Check sheet for the modelled part. Datum: model origin and axes. Units: mm. A direction names the side the tool comes from. Give positions to 0.01 mm unless a question says otherwise; leave off trailing zeros. Loops run counter-clockwise (first coordinate to the right, second up) from the corner with the lowest first, then second, coordinate; pieces in that order, holes last. Notation, with made-up numbers: M 28.25,36 L 37.25,36 A9 ccw 37.25,51 Z; hole C -12,-37 d6. An arc over 180 degrees is marked long. Use one line per item in the form item = value.
from build123d import *

# Parameters (mm, degrees)
SKETCH1_W                = 240
SKETCH1_H                = 240
BOSS_EXTRUDE1_DEPTH      = 20
CUT_EXTRUDE1_DEPTH       = 210.045449604
CUT_EXTRUDE1_DEPTH_BACK  = 210.045449604
SKETCH2_R                = 3.3
SKETCH3_R                = 5.5
CUT_EXTRUDE3_DEPTH       = 6.5
CUT_EXTRUDE4_DEPTH       = 210.045449604
CUT_EXTRUDE4_DEPTH_BACK  = 210.045449604
SKETCH4_R                = 6.75
SKETCH5_R                = 10
CUT_EXTRUDE6_DEPTH       = 13
CUT_EXTRUDE7_DEPTH       = 210.045449604
CUT_EXTRUDE7_DEPTH_BACK  = 210.045449604
SKETCH6_R                = 3.3
SKETCH7_R                = 5.5
CUT_EXTRUDE9_DEPTH       = 6.5
CUT_EXTRUDE10_DEPTH      = 210.045449604
CUT_EXTRUDE10_DEPTH_BACK = 210.045449604
SKETCH8_W                = 30
SKETCH8_H                = 260


with BuildPart() as part:
    # Sketch1 → Boss-Extrude1 (new body)
    with BuildSketch(Plane.XY):
        with Locations((0, -50)):
            Rectangle(SKETCH1_W, SKETCH1_H)
    extrude(amount=BOSS_EXTRUDE1_DEPTH)

    # Sketch2 → Cut-Extrude1 (cut, two sides: drawn at the far end of the back side and taken through both)
    with BuildSketch(Plane.XY.offset(-CUT_EXTRUDE1_DEPTH_BACK)):
        with Locations((-52, -63)):
            Circle(SKETCH2_R)
        with Locations((-52, 63)):
            Circle(SKETCH2_R)
        with Locations((52, -63)):
            Circle(SKETCH2_R)
        with Locations((52, 63)):
            Circle(SKETCH2_R)
    extrude(amount=CUT_EXTRUDE1_DEPTH + CUT_EXTRUDE1_DEPTH_BACK, mode=Mode.SUBTRACT)

    # Sketch3 → Cut-Extrude3 (cut)
    with BuildSketch(Plane.XY.offset(20)):
        with Locations((-52, -63)):
            Circle(SKETCH3_R)
        with Locations((-52, 63)):
            Circle(SKETCH3_R)
        with Locations((52, -63)):
            Circle(SKETCH3_R)
        with Locations((52, 63)):
            Circle(SKETCH3_R)
    extrude(amount=-CUT_EXTRUDE3_DEPTH, mode=Mode.SUBTRACT)

    # Sketch4 → Cut-Extrude4 (cut, two sides: drawn at the far end of the back side and taken through both)
    with BuildSketch(Plane.XY.offset(-CUT_EXTRUDE4_DEPTH_BACK)):
        with Locations((-20, -90)):
            Circle(SKETCH4_R)
        with Locations((20, -90)):
            Circle(SKETCH4_R)
    extrude(amount=CUT_EXTRUDE4_DEPTH + CUT_EXTRUDE4_DEPTH_BACK, mode=Mode.SUBTRACT)

    # Sketch5 → Cut-Extrude6 (cut)
    with BuildSketch(Plane.XY):
        with Locations((-20, -90)):
            Circle(SKETCH5_R)
        with Locations((20, -90)):
            Circle(SKETCH5_R)
    extrude(amount=CUT_EXTRUDE6_DEPTH, mode=Mode.SUBTRACT)

    # Sketch6 → Cut-Extrude7 (cut, two sides: drawn at the far end of the back side and taken through both)
    with BuildSketch(Plane.XY.offset(-CUT_EXTRUDE7_DEPTH_BACK)):
        with Locations((-46, -130)):
            Circle(SKETCH6_R)
        with Locations((-46, -155)):
            Circle(SKETCH6_R)
        with Locations((46, -130)):
            Circle(SKETCH6_R)
        with Locations((46, -155)):
            Circle(SKETCH6_R)
    extrude(amount=CUT_EXTRUDE7_DEPTH + CUT_EXTRUDE7_DEPTH_BACK, mode=Mode.SUBTRACT)

    # Sketch7 → Cut-Extrude9 (cut)
    with BuildSketch(Plane.XY):
        with Locations((-46, -130)):
            Circle(SKETCH7_R)
        with Locations((-46, -155)):
            Circle(SKETCH7_R)
        with Locations((46, -130)):
            Circle(SKETCH7_R)
        with Locations((46, -155)):
            Circle(SKETCH7_R)
    extrude(amount=CUT_EXTRUDE9_DEPTH, mode=Mode.SUBTRACT)

    # Sketch8 → Cut-Extrude10 (cut, two sides: drawn at the far end of the back side and taken through both)
    with BuildSketch(Plane.XY.offset(-CUT_EXTRUDE10_DEPTH_BACK)):
        with Locations((-115, -50)):
            Rectangle(SKETCH8_W, SKETCH8_H)
        with Locations((115, -50)):
            Rectangle(SKETCH8_W, SKETCH8_H)
    extrude(amount=CUT_EXTRUDE10_DEPTH + CUT_EXTRUDE10_DEPTH_BACK, mode=Mode.SUBTRACT)


solid = part.part
1) Section check B-B (z = 3.75). State how many separate pieces and enclosed holes the cut face has, then the cut area to 3 significant figures.
Evaluation:
separate_pieces = 1
enclosed_holes = 10
area = 46,900 mm^2
2) Depth check by flat-ended pin: pin 1 Ø9 at (x, y) = (-45.5, -155.5) entering from -Z; pin 2 Ø3.5 at (x, y) = (-51, -64) entering from +Z; pin 3 Ø6 at (x, y) = (-24, -85.5) entering from -Z; pin 4 Ø3.5 at (x, y) = (-53, 65.5) entering from +Z. Enter the tip coordinate at first touch or a pass-through.
Evaluation:
pin_1 = 6.5
pin_2 = through
pin_3 = 13
pin_4 = 13.5
3) Release check for a two-part mould opening along Y. For faces 1 (the face through (-1, 70, 10)), 2 (the face through (18.54, -96.59, 16.45)), 3 (the face through (-52, -67, 13.5)), 4 (the face through (-1, -48, 0)) record: pulls with the +Y half, pulls with the -Y half, needs draft (parallel to the pull), parting line crosses it, or undercut.
Evaluation:
face_1 = pulls with the +Y half
face_2 = undercut
face_3 = undercut
face_4 = needs draft
4) Section check A-A (y = -90). Record the cut outline in (x, z).
Evaluation:
outline = M -100,0 L -30,0 L -30,13 L -26.75,13 L -26.75,20 L -100,20 Z; M -13.25,13 L -10,13 L -10,0 L 10,0 L 10,13 L 13.25,13 L 13.25,20 L -13.25,20 Z; M 26.75,13 L 30,13 L 30,0 L 100,0 L 100,20 L 26.75,20 Z
5) Section check C-C (x = -20). Record the cut outline in (y, z), then the cut area to 3 significant figures.
Evaluation:
outline = M -170,0 L -100,0 L -100,13 L -96.75,13 L -96.75,20 L -170,20 Z; M -83.25,13 L -80,13 L -80,0 L 70,0 L 70,20 L -83.25,20 Z
area = 4,450 mm^2
6) Set-up check for faces 5 (the face through (49.57, 65.23, 6.66)), 6 (the face through (47.95, -59.28, 16.8)), 7 (the face through (-46.716, -124.547, 3.204)): record each of +Z, -Z, +X, -X, +Y, -Y from which the full face is reachable in a straight line by a thin tool's end or side.
Evaluation:
face_5 = +Z, -Z
face_6 = +Z
face_7 = -Z
7) Section check D-D (y = -155). Record the cut outline in (x, z).
Evaluation:
outline = M -100,0 L -51.5,0 L -51.5,6.5 L -49.3,6.5 L -49.3,20 L -100,20 Z; M -42.7,6.5 L -40.5,6.5 L -40.5,0 L 40.5,0 L 40.5,6.5 L 42.7,6.5 L 42.7,20 L -42.7,20 Z; M 49.3,6.5 L 51.5,6.5 L 51.5,0 L 100,0 L 100,20 L 49.3,20 Z
8) Scan lines: line 1 (Y direction, x = -52, z = 16); line 2 (X direction, y = 63, z = 5.75); line 3 (Y direction, x = 46, z = 13.25). Record each from-to range of solid material in increasing order.
Evaluation:
line_1 = -170 to -68.5, -57.5 to 57.5, 68.5 to 70
line_2 = -100 to -55.3, -48.7 to 48.7, 55.3 to 100
line_3 = -170 to -158.3, -151.7 to -133.3, -126.7 to 70
